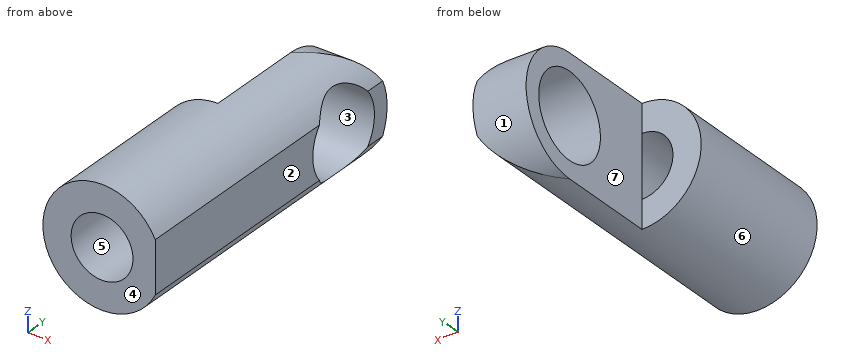
Autodesk Inventor part; units mm, degrees
ref_plane "YZ Plane" through (0, 0, 0) normal (1, 0, 0) x (0, 1, 0)
ref_plane "XZ Plane" through (0, 0, 0) normal (0, 1, 0) x (-1, 0, 0)
ref_plane "XY Plane" through (0, 0, 0) normal (0, 0, 1) x (1, 0, 0)
sketch "Sketch1" plane through (0, 0, 0) normal (0, 1, 0) x (-1, 0, 0)
  circle A0 centre (0, 0) radius 4.7625
  dimension "d0" = 9.525
extrude "Extrusion1" add sketch "Sketch1" along normal blind 12.7
sketch "Sketch2" plane through (0, 0, 0) normal (0, -1, 0) x (1, 0, 0)
  circle A0 centre (0, 0) radius 2.539
hole "Hole1" at (0, 0, 0) direction (0, 1, 0) diameter 4.9784 depth 19.05 tip angle 118
sketch "Sketch3" plane through (0, 12.7, 0) normal (0, 1, 0) x (1, 0, 0)
  circle A0 centre (0, 0) radius 4.7625
  circle A1 centre (0, 0) radius 4.7625
  line L0 (0, -4.7625) -> (0, 4.7625)
  dimension "d10" = 9.525
extrude "Extrusion2" add sketch "Sketch3" along normal blind 12.7 contours A0 L0 picked at (1.6786, -1.3984)
sketch "Sketch4" plane through (0, 12.7, -2.4892) normal (-1, 0, 0) x (0, 0, 1)
  line L0 (-2.2733, 0) -> (-2.2733, 12.7)
  line L1 (7.2517, 0) -> (7.2517, 12.7)
  line L2 (-2.2733, 0) -> (7.2517, 0)
  line L3 (7.2517, 0) -> (7.2517, 12.7)
  line L4 (7.2517, 12.7) -> (-2.2733, 12.7)
  line L5 (-2.2733, 12.7) -> (-2.2733, 0)
  arc A0 (7.2517, 7.9375) -> (-2.2733, 7.9375) centre (2.4892, 7.9375) ccw
  line L6 (7.2517, 12.7) -> (-2.2733, 12.7)
  line L7 (-2.2733, 7.9375) -> (-2.2733, 12.7)
  line L8 (-2.2733, 12.7) -> (7.2517, 12.7)
  line L9 (7.2517, 12.7) -> (7.2517, 7.9375)
  point P0 (2.4892, -12.7)
extrude "Extrusion3" cut sketch "Sketch4" against normal blind 12.7 contours L0 L4 A0 | L4 L1 A0
sketch "Sketch5" plane through (0, 12.7, -2.4892) normal (-1, 0, 0) x (0, 0, 1)
  arc A0 (7.2517, 7.9375) -> (-2.2733, 7.9375) centre (2.4892, 7.9375) ccw
  circle A1 centre (2.4892, 7.9375) radius 2.2013
  point P0 (2.4892, -12.7)
hole "Hole2" at (0, 20.6375, 0) direction (1, 0, 0) diameter 6.7564 depth 19.05 tip angle 118
sketch "Sketch6" plane through (0, 0, 0) normal (0, -1, 0) x (1, 0, 0)
  line L0 (0, 0) -> (4.7909, 0)
  line L1 (5.3024, 5.1468) -> (4.2794, 5.1468)
  line L2 (4.2794, 5.1468) -> (4.2794, -5.1468)
  line L3 (4.2794, -5.1468) -> (5.3024, -5.1468)
  line L4 (5.3024, -5.1468) -> (5.3024, 5.1468)
  line L5 (5.3024, 5.1468) -> (4.2794, -5.1468) construction
  line L6 (4.2794, 5.1468) -> (5.3024, -5.1468) construction
extrude "Extrusion4" cut sketch "Sketch6" against normal blind 25.4
properties part number "feet type 3 part 1" material "Stainless Steel"
Verification items for the finished model (mm, model axes). Face numbers are marked on the shaded views. A direction names the side the tool comes from. Give positions to 0.01 mm unless a question says otherwise; leave off trailing zeros. Write each loop counter-clockwise with the first axis right and the second up, starting at its lowest first coordinate (ties: lowest second). Pieces come first, ordered by that corner, then holes. Notation, with made-up numbers: (75.5, 50.5) -> (96.5, 50.5) arc R10 cw to (96.5, 62.5) -> close; hole circle Ø8 at (8.5, 21.5). An arc over 180 degrees is marked (long way). Use CSV: the item, a comma, the result in double quotes.
(1) Sectioned sample at D-D (x = 0.5). Record the cut outline in (y, z) (1 decimal).
Derived:
outline,"(0, -4.7) -> (21.1, -4.7) arc R4.8 ccw to (21.1, 4.7) -> (0, 4.7) -> (0, 2.4) -> (12.7, 2.4) -> (12.7, -2.4) -> (0, -2.4) -> close; hole circle Ø6.8 at (20.6, 0)"
(2) Sectioned sample at A-A (z = 0). Record the cut outline in (x, y), plus the area to 3 significant figures.
Derived:
outline,"(-4.76, 0) -> (-2.49, 0) -> (-2.49, 12.7) -> (-4.76, 12.7) -> close; (0, 12.7) -> (2.49, 12.7) -> (2.49, 0) -> (4.28, 0) -> (4.28, 17.26) -> (0, 17.26) -> close; (0, 24.02) -> (4.28, 24.02) -> (4.28, 25.4) -> (0, 25.4) -> close"
area,"77.0 mm^2"
(3) Sectioned sample at B-B (x = -1.25). Record the cut outline in (y, z).
Derived:
outline,"(0, -4.6) -> (12.7, -4.6) -> (12.7, -2.15) -> (0, -2.15) -> close; (0, 2.15) -> (12.7, 2.15) -> (12.7, 4.6) -> (0, 4.6) -> close"
(4) Material ranges on L1, parallel to Z at x = 0, y = 8.75; L2, parallel to X at y = 7.25, z = 0; L3, parallel to Y at x = -3, z = 1, recorded low to high.
Derived:
L1,"z = -4.76 to -2.49, 2.49 to 4.76"
L2,"x = -4.76 to -2.49, 2.49 to 4.28"
L3,"y = 0 to 12.7"
(5) Go/stop test with flat-tipped pins: pin 1 (2 mm diameter, centred on x = 1, z = 0.5, fed in from -Y); pin 2 (1.5 mm diameter, centred on x = -1.5, z = 3, fed in from -Y); pin 3 (4 mm diameter, centred on x = -3, z = -1.5, fed in from +Y); pin 4 (5 mm diameter, centred on y = 21.5, z = 1.5, fed in from -X). Record where each tip stops, or that it passes through.
Derived:
pin 1,"stops at y = 12.7"
pin 2,"stops at y = 0"
pin 3,"stops at y = 12.7"
pin 4,"stops at x = 0"
(6) Set-up check for the marked faces 5, 6 and 7: record each of +Z, -Z, +X, -X, +Y, -Y from which the full face is reachable in a straight line by a thin tool's end or side.
Derived:
face 5,"-Y"
face 6,"+Y, -Y"
face 7,"+Z, -Z, -X, +Y"
(7) Sectioned sample at C-C (y = 23). Record the cut outline in (x, z) (1 decimal), plus the area to 3 significant figures.
Derived:
outline,"(0, -4.1) -> (2.4, -4.1) arc R4.8 ccw to (4.1, -2.4) -> (0, -2.4) -> close; (0, 2.4) -> (4.1, 2.4) arc R4.8 ccw to (2.4, 4.1) -> (0, 4.1) -> close"
area,"11.7 mm^2"
(8) Release check for a two-part mould opening along Y. For the marked faces 1, 2, 3 and 4 record: +Y half, -Y half, draft (parallel to the pull), parting line (faces both ways), or undercut.
Derived:
face 1,"+Y half"
face 2,"draft"
face 3,"undercut"
face 4,"-Y half"
